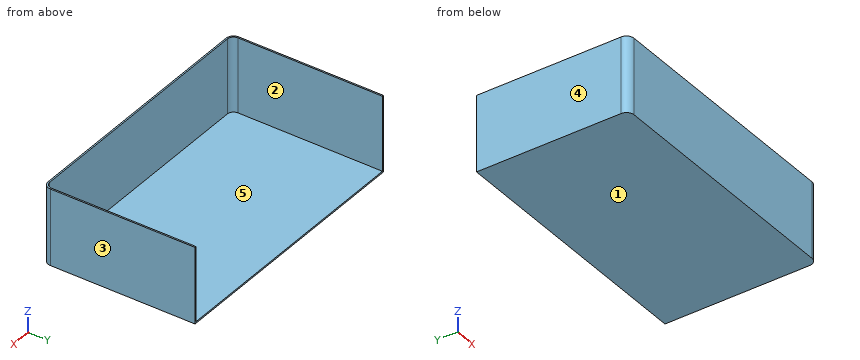
from build123d import *

# Parameters (mm, degrees)
SKETCH_1_W      = 350
SKETCH_1_H      = 200
EXTRUDE_1_DEPTH = 100
FILLET_1_R      = 10
SHELL_1_T       = -2


with BuildPart() as part:
    # 草图1 → 凸台-拉伸1 (new body)
    with BuildSketch(Plane.XY):
        Rectangle(SKETCH_1_W, SKETCH_1_H)
    extrude(amount=EXTRUDE_1_DEPTH)

    # 圆角1
    fillet_1_edges = [part.edges().sort_by_distance(p)[0] for p in [
        (175, -100, 50),
        (-175, -100, 50),
    ]]
    fillet(fillet_1_edges, radius=FILLET_1_R)

    # 抽壳1
    shell_1_openings = [part.faces().sort_by_distance(p)[0] for p in [
        (0, 0.059982012, 100),
        (0, 100, 50),
    ]]
    offset(amount=SHELL_1_T, openings=shell_1_openings, kind=Kind.INTERSECTION)


solid = part.part
For this review, take the finished solid that the model builds, in its own axes (mm). Face numbers are marked on the shaded views. A direction names the side the tool comes from. Give positions to 0.01 mm unless a question says otherwise; leave off trailing zeros. Order: outer loops, then holes, each group sorted by start corner. A loop starts at its lowest first (then second) coordinate and runs counter-clockwise, first axis right, second up. Notation, with made-up numbers: (-26.75, -34) - (28.25, -34) arc R18 cw to (28.25, -7) - close; hole circle Ø4 at (54.25, 20.25). An arc over 180 degrees is marked (long way). Answer as a JSON object with one key per item and string values. Group by question number.
Item 1: Draft analysis for pull direction X (two halves, no side actions). For the marked faces 3, 4 and 5, state which applies: pulls with the +X half, pulls with the -X half, needs draft (parallel to the pull), parting line crosses it, or undercut.
Item 2: Clearance check with flat-ended pins moving along their axes: pin 1 Ø8 at (x, y) = (30, -77) entering from +Z; pin 2 Ø8 at (x, z) = (-5.5, 23) entering from +Y. State where each tip first meets the part, or that it passes through.
Item 3: Take a section at A-A on y = 31. Give the boundary of the cut face in (x, z).
Item 4: Machinability: for the marked faces 1 and 2, which of the approach directions +Z, -Z, +X, -X, +Y, -Y give a long, thin tool a straight path to every point of the face, cutting with its end or side? Answer none if there is none.
Item 5: Take a section at C-C on x = -67. Give the boundary of the cut face in (y, z), and give its area (3 significant figures).
Item 6: Wall thickness on line 1 along X through (y, z) = (-72, 50.5); line 2 along Y through (x, z) = (83.5, 17); line 3 along Z through (x, y) = (157.5, -83): over which ranges is each line inside the solid? List them lowest first.
Item 7: Take a section at B-B on z = 47. Give the boundary of the cut face in (x, y), and give its area (3 significant figures).
Reported:
{
 "1": {"face 3": "pulls with the +X half", "face 4": "pulls with the -X half", "face 5": "undercut"},
 "2": {"pin 1": "z = 2", "pin 2": "y = -98"},
 "3": {"outline": "(-175, 0) - (175, 0) - (175, 100) - (173, 100) - (173, 2) - (-173, 2) - (-173, 100) - (-175, 100) - close"},
 "4": {"face 1": "-Z, +X, -X, +Y, -Y", "face 2": "+Z, +Y"},
 "5": {"outline": "(-100, 0) - (100, 0) - (100, 2) - (-98, 2) - (-98, 100) - (-100, 100) - close", "area": "596 mm^2"},
 "6": {"line 1": "-175 to -173, 173 to 175", "line 2": "-100 to -98", "line 3": "0 to 2"},
 "7": {"outline": "(-175, -90) arc R10 ccw to (-165, -100) - (165, -100) arc R10 ccw to (175, -90) - (175, 100) - (173, 100) - (173, -90) arc R8 cw to (165, -98) - (-165, -98) arc R8 cw to (-173, -90) - (-173, 100) - (-175, 100) - close", "area": "1,480 mm^2"}
}
